from build123d import *

# Parameters (mm, degrees)
F1_DEPTH = 5
F2_R     = 4.99999


# Not quite as in the source:
# - a fillet or chamfer is up to 0.001 mm smaller than in the source, because OpenCascade refuses the exact size
# - a feature of the source that left no trace in its solid (it failed there, or was rolled back) is left out


with BuildPart() as f1:
    # F0 (on Top) → F1 (new body)
    with BuildSketch(Plane.XY):
        with BuildLine():
            ThreePointArc((-21.6506350946, -12.5), (0, -18.3012701892), (21.6506350946, -12.5))
            ThreePointArc((21.6506350946, -12.5), (15.8493649054, 9.1506350946), (0, 25))
            ThreePointArc((0, 25), (-15.8493649054, 9.1506350946), (-21.6506350946, -12.5))
        make_face()
    extrude(amount=F1_DEPTH)

    # F2 (radius 5 in the source; OpenCascade refuses exactly that, so slightly less here)
    f2_edges = [f1.edges().sort_by_distance(p)[0] for p in [
        (-15.849365, 9.150635, 5),
        (0, -18.30127, 5),
        (15.849365, 9.150635, 5),
    ]]
    fillet(f2_edges, radius=F2_R)


solid = f1.part
Input: part model. Units: mm. Frame: model coordinates. Coordinates: 2 decimals unless noted, no trailing zeros. Loops run counter-clockwise (first coordinate to the right, second up) from the corner with the lowest first, then second, coordinate; pieces in that order, holes last. Notation, with made-up numbers: (72.5, 50.25) -> (77.5, 50.25) arc R7 ccw to (77.5, 58.25) -> close; hole circle Ø4 at (-37.75, 0). An arc over 180 degrees is marked (long way). One line per item, written item: value.
(1) Cut plane A-A (z = 1.7). Output: boundary loops of the cut face in (x, y), then the cut area to 3 significant figures.
Answer below:
outline: (-21.35, -12.33) arc R43 ccw to (21.35, -12.33) arc R43 ccw to (0, 24.66) arc R43 ccw to start
area: 1,280 mm2
(2) Ray query, line 1 along Y through (x, z) = (10.5, 3.4); line 2 along Z through (x, y) = (13.5, -12); line 3 along X through (y, z) = (-6, 4.1). Return the intervals inside material, ascending.
Answer below:
line 1: y = -15.63 to 14.47
line 2: z = 0 to 4.88
line 3: x = -19 to 19
(3) Pin query (flat end, axial travel): pin 1 Ø1.5 at (x, z) = (-0.5, 2) entering from +Y; pin 2 Ø2 at (x, y) = (-15, 3.5) entering from +Z; pin 3 Ø1.5 at (y, z) = (-11.5, 3) entering from -X. Return the tip coordinate at first contact, or that it passes through.
Answer below:
pin 1: stops at y = 24.75
pin 2: stops at z = 4.95
pin 3: stops at x = -21.1
